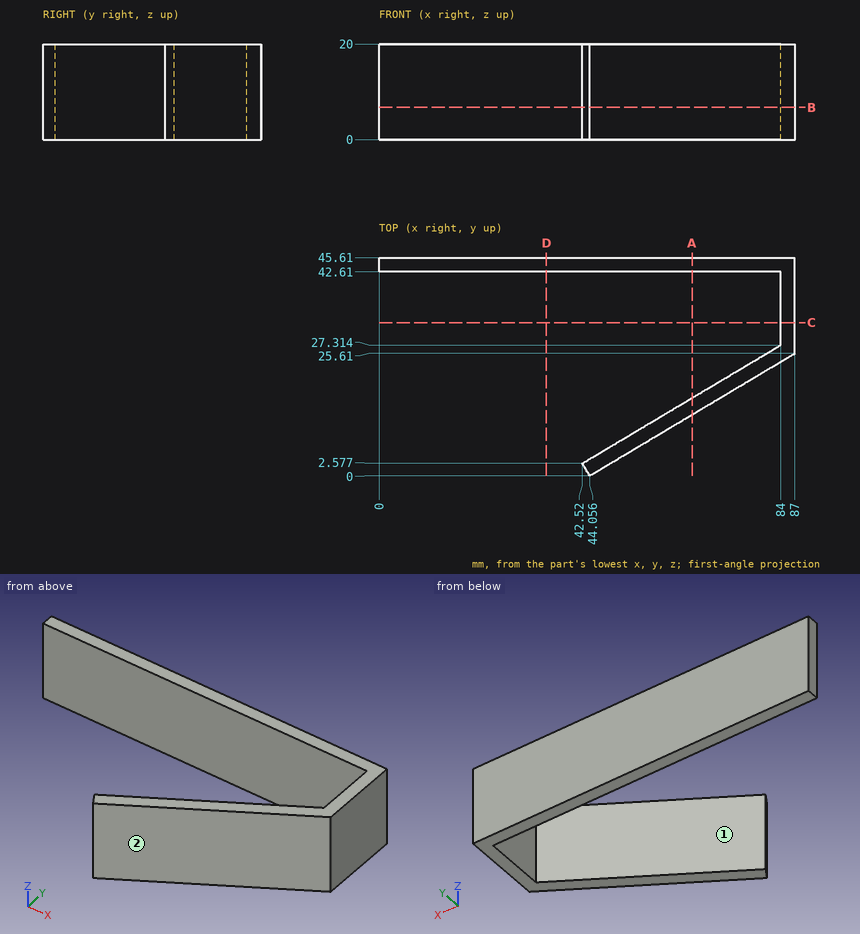
Verification items for this drawing (mm, ordinates from the low corner). A direction names the side the tool comes from. Coordinates: 2 decimals unless noted, no trailing zeros. Loops run counter-clockwise (first coordinate to the right, second up) from the corner with the lowest first, then second, coordinate; pieces in that order, holes last. Notation, with made-up numbers: (-9, 4.5) -> (30, 4.5) arc R15 ccw to (30, 30.5) -> close; hole circle Ø6 at (62, 39.5). An arc over 180 degrees is marked (long way). Put each result on its own line as item: value.
1. Section check C-C, the plane y = 32. Record the boundary of the cut face in (x, z).
Result set:
outline: (84, 0) -> (87, 0) -> (87, 20) -> (84, 20) -> close
2. Gauge pin test, flat ends, axial feed: P1, Ø6, axis at y = 37.5, z = 11, coming from the -X side; P2, Ø8, axis at y = 7, z = 5, coming from the -X side; P3, Ø1.5, axis at y = 22, z = 7.5, coming from the -X side (1 decimal). Record the tip position at first contact, or that the pin passes through.
Result set:
P1: stops at x = 84
P2: stops at x = 43.23
P3: stops at x = 73.8
3. Tool access check on the marked faces 1 and 2. Record the directions out of +Z, -Z, +X, -X, +Y, -Y that give a thin tool (end or side, any length) a straight path to the whole face; none if there is none.
Result set:
face 1: +Z, -Z, -X
face 2: +Z, -Z, +X, -Y
4. Section check B-B, the plane z = 6.75. Record the boundary of the cut face in (x, y), then the cut area to 3 significant figures.
Result set:
outline: (0, 42.61) -> (84, 42.61) -> (84, 27.31) -> (42.52, 2.58) -> (44.06, 0) -> (87, 25.61) -> (87, 45.61) -> (0, 45.61) -> close
area: 457 mm^2
5. Section check A-A, the plane x = 65.5. Record the boundary of the cut face in (y, z).
Result set:
outline: (12.79, 0) -> (16.28, 0) -> (16.28, 20) -> (12.79, 20) -> close; (42.61, 0) -> (45.61, 0) -> (45.61, 20) -> (42.61, 20) -> close
6. Section check D-D, the plane x = 35. Record the boundary of the cut face in (y, z), then the cut area to 3 significant figures.
Result set:
outline: (42.61, 0) -> (45.61, 0) -> (45.61, 20) -> (42.61, 20) -> close
area: 60.0 mm^2
7. Thickness scan on line 1 (X direction, y = 42.5, z = 12); line 2 (Y direction, x = 23.5, z = 18.75); line 3 (Y direction, x = 50, z = 10.75) (1 decimal). Record the ranges inside material, lowest first.
Result set:
line 1: x = 84 to 87
line 2: y = 42.61 to 45.61
line 3: y = 3.5 to 7, 42.6 to 45.6
